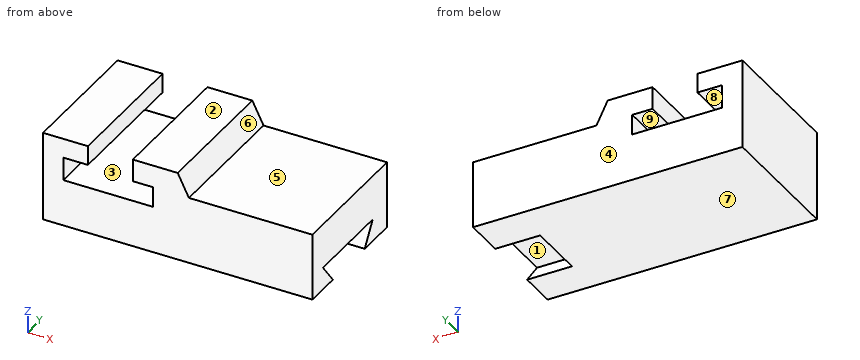
```python
from build123d import *

# Parameters (mm, degrees)
F1_DEPTH = 76.2
F3_DEPTH = 25.4


with BuildPart() as f1:
    # F0 (on Front) → F1 (new body)
    with BuildSketch(Plane.XZ):
        Polygon((-53.467005, 35.687), (-53.467005, -15.113), (98.932995, -15.113), (98.932995, 22.987), (29.082995, 22.987), (22.732995, 35.687), (-2.667005, 35.687), (-2.667005, 22.987), (8.837793, 22.987), (8.837793, 11.473469), (-41.962207, 11.473469), (-41.962207, 24.681469), (-28.067005, 24.681469), (-28.067005, 35.687), align=None)
    extrude(amount=F1_DEPTH)

    # F2 (on face) → F3 (cut)
    with BuildSketch(Plane.YZ.offset(98.932995)):
        Polygon((-14.604999, -2.413), (-65.404999, -2.413), (-55.245001, -15.113), (-22.732999, -15.113), align=None)
    extrude(amount=-F3_DEPTH, mode=Mode.SUBTRACT)


solid = f1.part
```
Check sheet for the modelled part. Datum: model origin and axes. Units: mm. Face numbers are marked on the shaded views. A direction names the side the tool comes from. Give positions to 0.01 mm unless a question says otherwise; leave off trailing zeros. Write each loop counter-clockwise with the first axis right and the second up, starting at its lowest first coordinate (ties: lowest second). Pieces come first, ordered by that corner, then holes. Notation, with made-up numbers: (36, -29) - (70, -29) arc R20 cw to (70, -23) - close; hole circle Ø8 at (-1, -8). An arc over 180 degrees is marked (long way). Answer as a JSON object with one key per item and string values. Group by question number.
1) Sectioned sample at D-D (x = 71.5). Record the cut outline in (y, z), then the cut area to 3 significant figures.
2) Sectioned sample at A-A (x = 88). Record the cut outline in (y, z) (3 decimals), then the cut area to 3 significant figures.
3) Sectioned sample at C-C (z = -9.5). Record the cut outline in (x, y), then the cut area to 3 significant figures.
4) Release check for a two-part mould opening along X. For the marked faces 6, 7, 8 and 9 record: pulls with the +X half, pulls with the -X half, needs draft (parallel to the pull), parting line crosses it, or undercut.
5) Thickness scan on probe 1 along X at (y, z) = (-41.5, 15.5); probe 2 along Z at (x, y) = (8.5, -61.5); probe 3 along Z at (x, y) = (-37, -66.5). Record the ranges inside material, lowest first. Write a range as from..to.
6) Depth check by flat-ended pin: P1, Ø2, axis at x = 23.5, y = -24.5, coming from the +Z side; P2, Ø4, axis at y = -36.5, z = -8, coming from the +X side; P3, Ø1.5, axis at x = 53, y = -23, coming from the +Z side; P4, Ø15, axis at x = -18.5, y = -26.5, coming from the +Z side. Enter the tip coordinate at first touch or a pass-through.
7) Access from +Z, -Z, +X, -X, +Y, -Y to the whole of each face (thin tool, end or side, straight path). Record for the marked faces 1, 2, 3, 4 and 5.
8) Sectioned sample at B-B (y = -24.5). Record the cut outline in (x, z), then the cut area to 3 significant figures.
Geometry results:
{
 "1": {"outline": "(-76.2, -15.11) - (0, -15.11) - (0, 22.99) - (-76.2, 22.99) - close", "area": "2,900 mm^2"},
 "2": {"outline": "(-76.2, -15.113) - (-55.245, -15.113) - (-65.405, -2.413) - (-14.605, -2.413) - (-22.733, -15.113) - (0, -15.113) - (0, 22.987) - (-76.2, 22.987) - close", "area": "2,370 mm^2"},
 "3": {"outline": "(-53.47, -76.2) - (98.93, -76.2) - (98.93, -59.74) - (73.53, -59.74) - (73.53, -19.14) - (98.93, -19.14) - (98.93, 0) - (-53.47, 0) - close", "area": "10,600 mm^2"},
 "4": {"face 6": "pulls with the +X half", "face 7": "needs draft", "face 8": "undercut", "face 9": "undercut"},
 "5": {"probe 1": "x = -53.47..-41.96, 8.84..98.93", "probe 2": "z = -15.11..11.47, 22.99..35.69", "probe 3": "z = -15.11..11.47, 24.68..35.69"},
 "6": {"P1": "stops at z = 35.69", "P2": "stops at x = 73.53", "P3": "stops at z = 22.99", "P4": "stops at z = 11.47"},
 "7": {"face 1": "+X", "face 2": "+Z, +X, -X, +Y, -Y", "face 3": "+Y, -Y", "face 4": "+Z, -Z, +X, -X, +Y", "face 5": "+Z, +X, +Y, -Y"},
 "8": {"outline": "(-53.47, -15.11) - (73.53, -15.11) - (73.53, -2.41) - (98.93, -2.41) - (98.93, 22.99) - (29.08, 22.99) - (22.73, 35.69) - (-2.67, 35.69) - (-2.67, 22.99) - (8.84, 22.99) - (8.84, 11.47) - (-41.96, 11.47) - (-41.96, 24.68) - (-28.07, 24.68) - (-28.07, 35.69) - (-53.47, 35.69) - close", "area": "5,560 mm^2"}
}
